Autodesk Inventor part; units mm, degrees
ref_plane "YZ Plane" through (0, 0, 0) normal (1, 0, 0) x (0, 1, 0)
ref_plane "XZ Plane" through (0, 0, 0) normal (0, 1, 0) x (-1, 0, 0)
ref_plane "XY Plane" through (0, 0, 0) normal (0, 0, 1) x (1, 0, 0)
sketch "スケッチ1" plane through (0, 0, 0) normal (0, 0, 1) x (1, 0, 0)
  line L0 (-30.25, 14.5) -> (30.25, 14.5)
  line L1 (30.25, 14.5) -> (30.25, -14.5)
  line L2 (30.25, -14.5) -> (-30.25, -14.5)
  line L3 (-30.25, -14.5) -> (-30.25, 14.5)
  line L4 (-25.25, 11.5) -> (25.25, 11.5) construction
  line L5 (25.25, 11.5) -> (25.25, -11.5) construction
  line L6 (25.25, -11.5) -> (-25.25, -11.5) construction
  line L7 (-25.25, -11.5) -> (-25.25, 11.5) construction
  line L8 (25.25, 11.5) -> (-25.25, -11.5) construction
  line L9 (-25.25, -9.8518) -> (-25.25, 11.5)
  line L10 (-25.25, 11.5) -> (21.631, 11.5)
  line L11 (21.631, 11.5) -> (-25.25, -9.8518)
  line L12 (-21.631, -11.5) -> (25.25, -11.5)
  line L13 (25.25, -11.5) -> (25.25, 9.8518)
  line L14 (25.25, 9.8518) -> (-21.631, -11.5)
  line L15 (-30.25, 12) -> (30.25, 12) construction
  line L16 (30.25, -12) -> (-30.25, -12) construction
  line L17 (30.25, 12) -> (30.25, -12) construction
  point P0 (0, 0)
  point P1 (0, 11.5)
  point P2 (0, 14.5)
  point P3 (25.25, 0)
  point P4 (30.25, 0)
  dimension "d0" = 5
  dimension "d1" = 3
  dimension "d2" = 1.5
  dimension "d3" = 24
  dimension "d4" = 2.5
  dimension "d16" = 60.5
extrude "押し出し1" add sketch "スケッチ1" along normal blind 5
sketch "スケッチ2" plane through (30.25, -14.5, 0) normal (1, 0, 0) x (0, 0, -1)
  line L0 (0, 29) -> (-5, 29)
  line L1 (-5, 0) -> (-5, 29)
  line L2 (0, 14.5) -> (-5, 14.5) construction
  point P0 (-2.5, 2.5)
  point P1 (-2.5, 26.5)
  point P2 (-2.5, 29)
  dimension "d7" = 24
hole "穴1" at (30.25, -12, 2.5) at (30.25, 12, 2.5) direction (-1, 0, 0) diameter 2.459 depth 3
mirror "ミラー1" about plane through (0, 0, 0) normal (1, 0, 0) of "穴1"
fillet "フィレット1" radius 2 6 edges at (-21.631, -11.5, 2.5) (-25.25, -9.8518, 2.5) (25.25, 9.8518, 2.5) (25.25, -11.5, 2.5) (-25.25, 11.5, 2.5) (21.631, 11.5, 2.5)
equation "\"d3\" = d5_1"
properties part number "Link_back_diagonal" material "アルミニウム 2014-T4"
The listing builds one solid part. Answer for the finished solid, in the listing's coordinates (mm). A direction names the side the tool comes from. Coordinates: 2 decimals unless noted, no trailing zeros. Order: outer loops, then holes, each group sorted by start corner. A loop starts at its lowest first (then second) coordinate and runs counter-clockwise, first axis right, second up.
Q1. A cutting plane is placed at B-B, the plane x = 24. Write down the section's boundary in (y, z).
Q2. A cutting plane is placed at A-A, the plane z = 2.5. State how many separate pieces and enclosed holes the cut face has, and give its area (3 significant figures).
Q3. A cutting plane is placed at C-C, the plane y = 4.5. Write down the section's boundary in (x, z), and give its area (3 significant figures).
Q4. Given P1, Ø1.5, axis at y = 12, z = 2.5, coming from the -X side; P2, Ø2, axis at y = 12, z = 2.5, coming from the +X side, each flat-ended and moving along its own axis, determine where each tip first touches the part or whether it passes through.
Q5. Consider line 1 (Y direction, x = 29.5, z = 2.5); line 2 (Z direction, x = 28, y = 12); line 3 (X direction, y = 6, z = 1). Determine where each line is inside the solid, lowest interval first.
Q6. For a pull along Y with two mould halves and no side action, classify faces 1 (the face through (0, 0, 0)), 2 (the face through (-24.356, -8.41, 2.535)) as pulls with the +Y half, pulls with the -Y half, needs draft (parallel to the pull), parting line crosses it, or undercut.
Q7. Which of the six approach directions +Z, -Z, +X, -X, +Y, -Y give full straight-line access (tool end or side, diameter ignored) to faces 3 (the face through (-25.25, 1, 2)), 4 (the face through (-27.25, -12, 2)), 5 (the face through (27.25, -12, 3))?
Answers follow:
1. outline: (-14.5, 0) - (-11.35, 0) - (-11.35, 5) - (-14.5, 5) - close; (8.6, 0) - (14.5, 0) - (14.5, 5) - (8.6, 5) - close
2. separate pieces: 1
2. enclosed holes: 2
2. area: 756 mm2
3. outline: (-30.25, 0) - (-25.25, 0) - (-25.25, 5) - (-30.25, 5) - close; (6.26, 0) - (13.5, 0) - (13.5, 5) - (6.26, 5) - close; (25.25, 0) - (30.25, 0) - (30.25, 5) - (25.25, 5) - close
3. area: 86.2 mm2
4. P1: stops at x = -27.25
4. P2: stops at x = 27.25
5. line 1: y = -14.5 to -13.23, -10.77 to 10.77, 13.23 to 14.5
5. line 2: z = 0 to 1.27, 3.73 to 5
5. line 3: x = -30.25 to -25.25, 9.55 to 16.79, 25.25 to 30.25
6. face 1: needs draft
6. face 2: undercut
7. face 3: +Z, -Z
7. face 4: -X
7. face 5: +X
